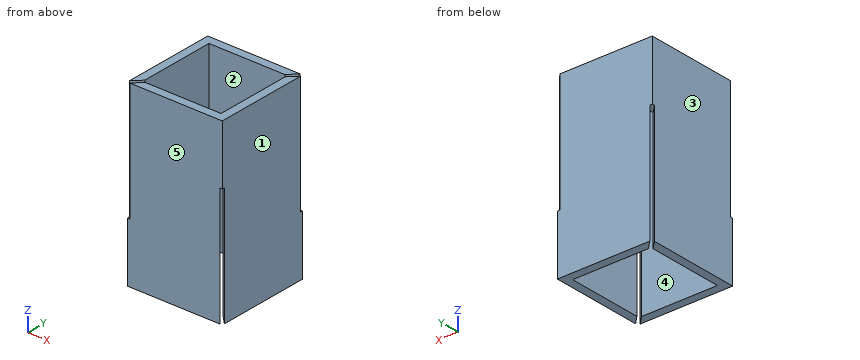
from build123d import *

# Parameters (mm, degrees)
F1_DEPTH = 15
F2_DEPTH = 5
F4_ANGLE = 90


with BuildPart() as f1:
    # F0 (on Top) → F1 (new body)
    with BuildSketch(Plane.XY):
        Polygon((-4, 4), (-4, -3.7878679656), (-3.3, -3.0878679656), (-3.3, 3.3), (3.0878679656, 3.3), (3.7878679656, 4), align=None)
        Polygon((-3.7878679656, -4), (4, -4), (4, 3.7878679656), (3.3, 3.0878679656), (3.3, -3.3), (-3.0878679656, -3.3), align=None)
    extrude(amount=F1_DEPTH)

    # F0 (on Top) → F2 (join)
    with BuildSketch(Plane.XY):
        Polygon((-4, -4), (-3.7878679656, -4), (-3.0878679656, -3.3), (-3.3, -3.3), (-3.3, -3.0878679656), (-4, -3.7878679656), align=None)
        Polygon((3.3, 3.0878679656), (4, 3.7878679656), (4, 4), (3.7878679656, 4), (3.0878679656, 3.3), (3.3, 3.3), align=None)
    extrude(amount=F2_DEPTH)


with BuildPart() as f3_1:
    # F3: instance of F1
    add(f1.part.mirror(Plane(origin=(-1.8837940264, 1.8837940264, 15), x_dir=(1, 0, 0), z_dir=(0, 0, 1))))


with BuildPart() as f3_1_1:
    # F4: moved
    add(f3_1.part.rotate(Axis((4, -4, 22.5), (0, 0, 1)), F4_ANGLE))


with BuildPart() as f3_1_2:
    # F5: moved
    add(f3_1_1.part.moved(Location((0, 8, -15))))


with BuildPart() as f1_1:
    add(f1.part)

    # F6: intersect F3_1
    add(f3_1_2.part, mode=Mode.INTERSECT)


solid = f1_1.part
CAD build for the part. Positions are in the model's coordinates, mm. Face numbers are marked on the shaded views. A direction names the side the tool comes from. Coordinates: 2 decimals unless noted, no trailing zeros. Write each loop counter-clockwise with the first axis right and the second up, starting at its lowest first coordinate (ties: lowest second). Pieces come first, ordered by that corner, then holes. Notation, with made-up numbers: (54.25, 11.5) - (74.25, 11.5) arc R19 cw to (74.25, 16.5) - close; hole circle Ø1 at (50, -0.5). An arc over 180 degrees is marked (long way). Use a Markdown table: item, result. Add a question column.
Item 1: Band-saw the part on B-B, the plane x = 0. Give the cut face in (y, z).
Item 2: Drill centre lines: L1, parallel to X at y = -2.5, z = 12.25; L2, parallel to Y at x = 3.5, z = 8. Where is each one in solid material? Low to high. Write a range as from..to.
Item 3: Band-saw the part on D-D, the plane z = 12. Give the cut face in (x, y), and give its area (3 significant figures).
Item 4: Band-saw the part on A-A, the plane z = 7. Give the cut face in (x, y), and give its area (3 significant figures).
Item 5: 3-axis set-ups, long thin cutter, end or side, ignore diameter. For the marked faces 1 and 2: which of +Z, -Z, +X, -X, +Y, -Y reach the whole face in a straight line?
Item 6: Mould opens along Y. For the marked faces 3, 4 and 5 say: pulls with the +Y half, pulls with the -Y half, needs draft (parallel to the pull), parting line crosses it, or undercut.
Numbers:
| question | item | result |
|---|---|---|
| 1 | outline | (-4, 0) - (-3.3, 0) - (-3.3, 15) - (-4, 15) - close; (3.3, 0) - (4, 0) - (4, 15) - (3.3, 15) - close |
| 2 | L1 | -4..-3.3, 3.3..4 |
| 2 | L2 | -4..-3.71, -3.29..3.29, 3.71..4 |
| 3 | outline | (-4, -3.79) - (-3.3, -3.09) - (-3.3, 3.3) - (3.09, 3.3) - (3.79, 4) - (-4, 4) - close; (-3.79, -4) - (4, -4) - (4, 3.79) - (3.3, 3.09) - (3.3, -3.3) - (-3.09, -3.3) - close |
| 3 | area | 19.8 mm2 |
| 4 | outline | (-4, -3.79) - (-3.3, -3.09) - (-3.3, 3.09) - (-4, 3.79) - close; (-3.79, -4) - (3.79, -4) - (3.09, -3.3) - (-3.09, -3.3) - close; (-3.79, 4) - (-3.09, 3.3) - (3.09, 3.3) - (3.79, 4) - close; (3.3, -3.09) - (4, -3.79) - (4, 3.79) - (3.3, 3.09) - close |
| 4 | area | 19.3 mm2 |
| 5 | face 1 | +Z, -Z, +X, +Y, -Y |
| 5 | face 2 | +Z, -Z |
| 6 | face 3 | needs draft |
| 6 | face 4 | undercut |
| 6 | face 5 | pulls with the -Y half |
